The drawing under review shows one solid part. Ordinate dimensions are in mm from its lowest x, y, z. Coordinates: 2 decimals unless noted, no trailing zeros. Loops run counter-clockwise (first coordinate to the right, second up) from the corner with the lowest first, then second, coordinate; pieces in that order, holes last. Notation, with made-up numbers: (5, -21) -> (10, -21) arc R20 ccw to (10, -14) -> close; hole circle Ø3 at (2, 58). An arc over 180 degrees is marked (long way). Use a Markdown table: item, result.
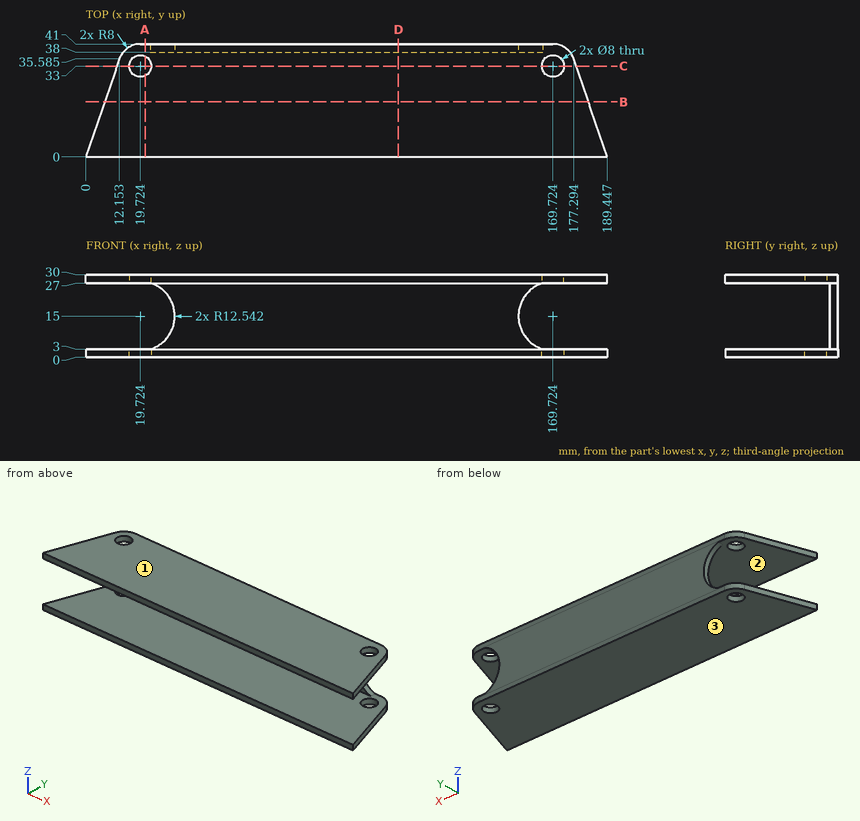
(1) For line 1 along Z through (x, y) = (97, 37); line 2 along Y through (x, z) = (59.5, 9.5); line 3 along X through (y, z) = (23.5, 27.25) (1 decimal), list the stretches that pass through material, from the lowest coordinate up.
Found:
| item | result |
|---|---|
| line 1 | z = 0 to 3, 27 to 30 |
| line 2 | y = 38 to 41 |
| line 3 | x = 8 to 181.4 |
(2) Take a section at B-B on y = 20. Write out the cut boundary in (x, z).
Found:
| item | result |
|---|---|
| outline | (6.83, 0) -> (182.62, 0) -> (182.62, 3) -> (6.83, 3) -> close; (6.83, 27) -> (182.62, 27) -> (182.62, 30) -> (6.83, 30) -> close |
(3) For pin 1 Ø7 at (x, z) = (120, 15.5) entering from -Y; pin 2 Ø5 at (y, z) = (6.5, 26) entering from +X, all flat-tipped, find the tip position at first contact; note any pin that passes through.
Found:
| item | result |
|---|---|
| pin 1 | stops at y = 38 |
| pin 2 | stops at x = 188.01 |
(4) Take a section at D-D on x = 113.5. Write out the cut boundary in (y, z), plus the area to 3 significant figures.
Found:
| item | result |
|---|---|
| outline | (0, 0) -> (41, 0) -> (41, 30) -> (0, 30) -> (0, 27) -> (38, 27) -> (38, 3) -> (0, 3) -> close |
| area | 318 mm^2 |
(5) Take a section at A-A on x = 21.5. Write out the cut boundary in (y, z) (1 decimal).
Found:
| item | result |
|---|---|
| outline | (0, 0) -> (29.4, 0) -> (29.4, 3) -> (0, 3) -> close; (0, 27) -> (29.4, 27) -> (29.4, 30) -> (0, 30) -> close; (36.6, 0) -> (41, 0) -> (41, 3) -> (36.6, 3) -> close; (36.6, 27) -> (41, 27) -> (41, 30) -> (36.6, 30) -> close |
(6) Take a section at C-C on y = 33. Write out the cut boundary in (x, z).
Found:
| item | result |
|---|---|
| outline | (11.27, 0) -> (15.72, 0) -> (15.72, 3) -> (11.27, 3) -> close; (11.27, 27) -> (15.72, 27) -> (15.72, 30) -> (11.27, 30) -> close; (23.72, 0) -> (165.72, 0) -> (165.72, 3) -> (23.72, 3) -> close; (23.72, 27) -> (165.72, 27) -> (165.72, 30) -> (23.72, 30) -> close; (173.72, 0) -> (178.18, 0) -> (178.18, 3) -> (173.72, 3) -> close; (173.72, 27) -> (178.18, 27) -> (178.18, 30) -> (173.72, 30) -> close |
(7) Mouldability with a two-part tool opening along Z and no side actions: class the marked faces 1, 2 and 3 as pulls with the +Z half, pulls with the -Z half, needs draft (parallel to the pull), parting line crosses it, or undercut.
Found:
| item | result |
|---|---|
| face 1 | pulls with the +Z half |
| face 2 | undercut |
| face 3 | pulls with the -Z half |
